Verification items for the finished model (mm, model axes). Coordinates: 2 decimals unless noted, no trailing zeros. Loops run counter-clockwise (first coordinate to the right, second up) from the corner with the lowest first, then second, coordinate; pieces in that order, holes last. Notation, with made-up numbers: (62, 65) -> (94, 65) arc R17 cw to (94, 78) -> close; hole circle Ø8 at (71, -13.75). An arc over 180 degrees is marked (long way). Answer as a JSON object with one key per item and string values. Group by question number.
Q1. Cross-section at A-A on x = 62. Record the boundary of the cut face in (y, z), and give its area (3 significant figures).
Q2. Scan lines: L1, parallel to Z at x = 12, y = 0.8; L2, parallel to X at y = 1.15, z = -10; L3, parallel to Z at x = 63.5, y = 0.9. Record each from-to range of solid material in increasing order.
Q3. Cross-section at B-B on z = -90. Record the boundary of the cut face in (x, y), and give its area (3 significant figures).
Q4. Release check for a two-part mould opening along X. For faces 1 (the cylindrical face through (62, 1, -92)), 2 (the flat face through (36, 0, -51)), 3 (the flat face through (0, 1, -49)), 4 (the cylindrical face through (10.526, 1.014, -11.352)) record: released by +X, released by -X, zero draft, split by the parting line, or undercut.
```python
from build123d import *

# Parameters (mm, degrees)
SKETCH1_W           = 74
SKETCH1_H           = 100
BOSS_EXTRUDE1_DEPTH = 2
FILLET1_R           = 2
SKETCH2_R           = 2
CUT_EXTRUDE1_DEPTH  = 3


with BuildPart() as part:
    # Sketch1 → Boss-Extrude1 (new body)
    with BuildSketch(Plane(origin=(0, 0, 0), x_dir=(1, 0, 0), z_dir=(0, 1, 0))):
        with Locations((37, 50)):
            Rectangle(SKETCH1_W, SKETCH1_H)
    extrude(amount=BOSS_EXTRUDE1_DEPTH)

    # Fillet1
    fillet1_edges = [part.edges().sort_by_distance(p)[0] for p in [
        (0, 1, -100),
        (74, 1, -100),
        (74, 1, 0),
        (0, 1, 0),
    ]]
    fillet(fillet1_edges, radius=FILLET1_R)

    # Sketch2 → Cut-Extrude1 (cut, through all)
    with BuildSketch(Plane(origin=(0, 2, 0), x_dir=(1, 0, 0), z_dir=(0, 1, 0))):
        with Locations((12, 90)):
            Circle(SKETCH2_R)
        with Locations((62, 90)):
            Circle(SKETCH2_R)
        with Locations((62, 10)):
            Circle(SKETCH2_R)
        with Locations((12, 10)):
            Circle(SKETCH2_R)
    extrude(amount=-CUT_EXTRUDE1_DEPTH, mode=Mode.SUBTRACT)


solid = part.part
```
Computed values:
{
 "1": {"outline": "(0, -100) -> (2, -100) -> (2, -92) -> (0, -92) -> close; (0, -88) -> (2, -88) -> (2, -12) -> (0, -12) -> close; (0, -8) -> (2, -8) -> (2, 0) -> (0, 0) -> close", "area": "184 mm²"},
 "2": {"L1": "z = -100 to -92, -88 to -12, -8 to 0", "L2": "x = 0 to 10, 14 to 60, 64 to 74", "L3": "z = -100 to -91.32, -88.68 to -11.32, -8.68 to 0"},
 "3": {"outline": "(0, 0) -> (10, 0) -> (10, 2) -> (0, 2) -> close; (14, 0) -> (60, 0) -> (60, 2) -> (14, 2) -> close; (64, 0) -> (74, 0) -> (74, 2) -> (64, 2) -> close", "area": "132 mm²"},
 "4": {"face 1": "undercut", "face 2": "zero draft", "face 3": "released by -X", "face 4": "undercut"}
}
